The drawing under review shows one solid part. Ordinate dimensions are in mm from its lowest x, y, z. A direction names the side the tool comes from. Round coordinates to 2 decimals unless told otherwise and drop trailing zeros. Order: outer loops, then holes, each group sorted by start corner. A loop starts at its lowest first (then second) coordinate and runs counter-clockwise, first axis right, second up. Notation, with made-up numbers: (38.25, 70.5) - (77.25, 70.5) arc R15 cw to (77.25, 84.5) - close; hole circle Ø5 at (54.25, 8.5). An arc over 180 degrees is marked (long way). One line per question, with ' | ' between items.
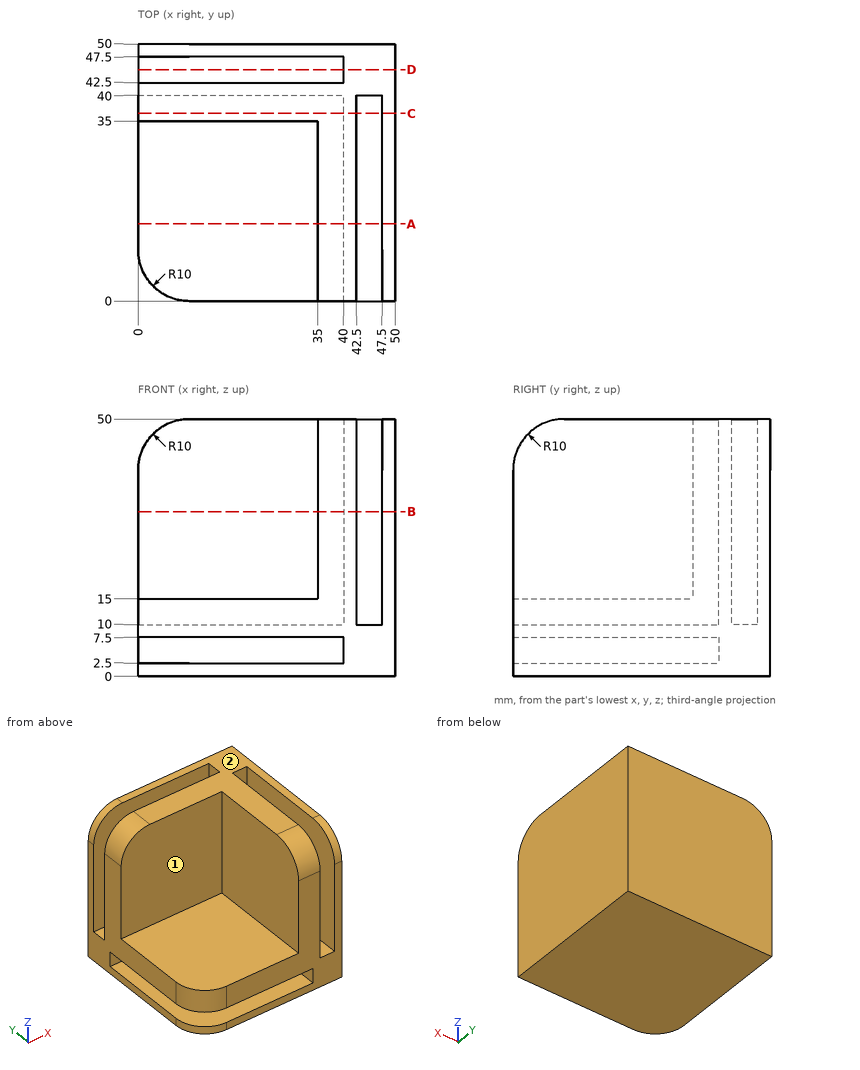
(1) We need section D-D on y = 45. State the section outline as (x, z) points.
Output values:
outline: (0, 0) - (50, 0) - (50, 50) - (40, 50) - (40, 10) - (0, 10) - close
(2) For probe 1 along X at (y, z) = (27.5, 17.5); probe 2 along Y at (x, z) = (38.5, 11), list the stretches that pass through material, from the lowest coordinate up. Write a range as [from, to].
Output values:
probe 1: [35, 42.5], [47.5, 50] | probe 2: [0, 42.5], [47.5, 50]
(3) Insertion check: pin 1 (2.5 mm diameter, centred on y = 21.5, z = 4, fed in from -X); pin 2 (17.5 mm diameter, centred on y = 23, z = 34.5, fed in from -X); pin 3 (2.5 mm diameter, centred on x = 46, y = 10.5, fed in from +Z). Each pin has a flat end and moves straight along its axis. Give the tip position at first contact, or say it passes through.
Output values:
pin 1: x = 40 | pin 2: x = 35 | pin 3: z = 10
(4) For the marked faces 1 and 2, list the 3-axis set-ups (+Z, -Z, +X, -X, +Y, -Y) from which the entire face can be reached by the end or side of a thin tool; tool diameter is ignored.
Output values:
face 1: +Z, -X, -Y | face 2: +Z, +X, -X, +Y, -Y
(5) We need section B-B on z = 32. State the section outline as (x, y) points, plus the area to 3 significant figures.
Output values:
outline: (0, 35) - (35, 35) - (35, 0) - (42.5, 0) - (42.5, 40) - (47.5, 40) - (47.5, 0) - (50, 0) - (50, 50) - (0, 50) - (0, 47.5) - (40, 47.5) - (40, 42.5) - (0, 42.5) - close | area: 875 mm^2
(6) We need section A-A on y = 15. State the section outline as (x, z) points.
Output values:
outline: (0, 0) - (50, 0) - (50, 50) - (47.5, 50) - (47.5, 10) - (42.5, 10) - (42.5, 50) - (35, 50) - (35, 15) - (0, 15) - (0, 7.5) - (40, 7.5) - (40, 2.5) - (0, 2.5) - close
(7) We need section C-C on y = 36.5. State the section outline as (x, z) points.
Output values:
outline: (0, 0) - (50, 0) - (50, 50) - (47.5, 50) - (47.5, 10) - (42.5, 10) - (42.5, 50) - (10, 50) arc R10 ccw to (0, 40) - (0, 7.5) - (40, 7.5) - (40, 2.5) - (0, 2.5) - close
